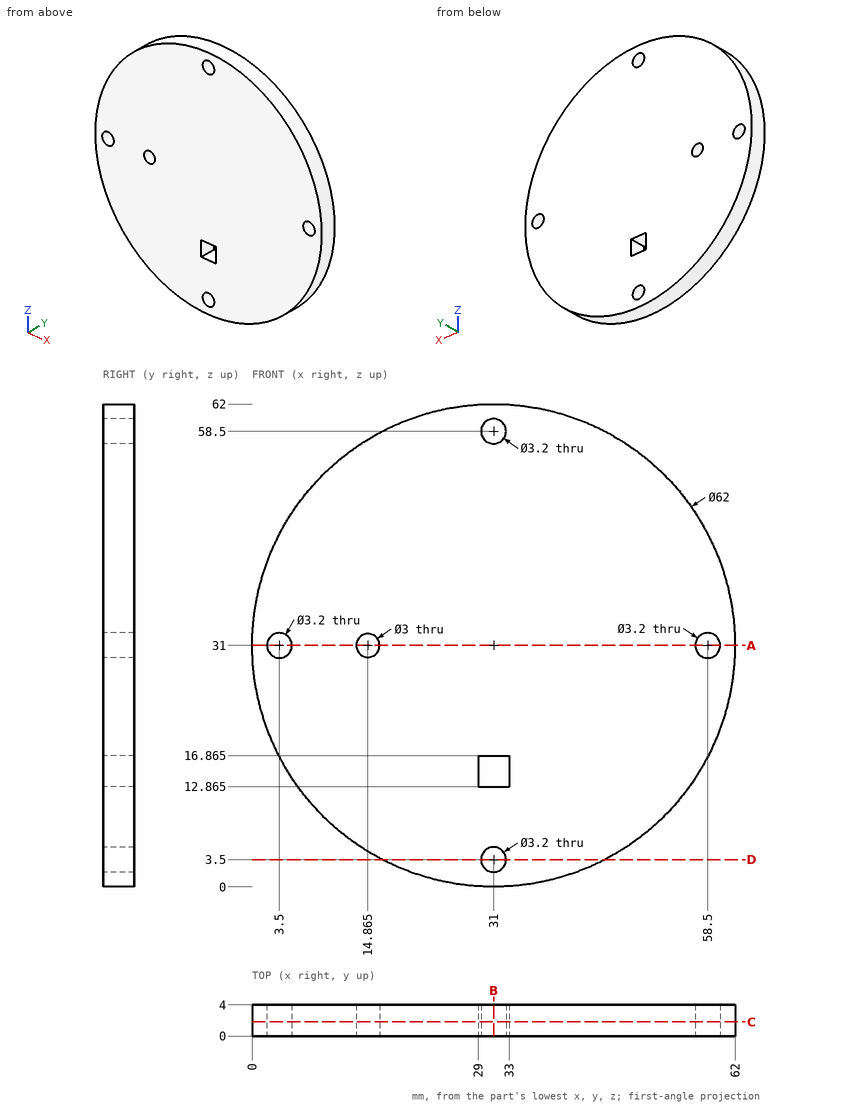
The drawing under review shows one solid part. Ordinate dimensions are in mm from its lowest x, y, z. Give positions to 0.01 mm unless a question says otherwise; leave off trailing zeros. Write each loop counter-clockwise with the first axis right and the second up, starting at its lowest first coordinate (ties: lowest second). Pieces come first, ordered by that corner, then holes.
1. Add section C-C, the plane y = 1.8. Write out the cut boundary in (x, z) (3 decimals).
2. Add section A-A, the plane z = 31. Write out the cut boundary in (x, y) (3 decimals).
3. Add section B-B, the plane x = 31. Write out the cut boundary in (y, z) (3 decimals).
4. Wall thickness on L1, parallel to X at y = 2.9, z = 31 (3 decimals); L2, parallel to X at y = 0.6, z = 16; L3, parallel to Z at x = 3.5, y = 1.45: over which ranges is each line inside the solid? List them lowest first.
5. Add section D-D, the plane z = 3.5. Write out the cut boundary in (x, y), plus the area to 3 significant figures.
6. For P1, Ø1, axis at x = 51.5, y = 3, coming from the -Z side; P2, Ø3, axis at x = 31, z = 58.5, coming from the +Y side; P3, Ø1.2, axis at x = 32, y = 1.5, coming from the +Z side; P4, Ø1, axis at x = 22, y = 3, coming from the -Z side, all flat-tipped, find the tip position at first contact; note any pin that passes through.
Worked answers:
1. outline: circle Ø62 at (31, 31); hole circle Ø3.2 at (3.5, 31); hole circle Ø3 at (14.865, 31); hole (29, 12.865) - (33, 12.865) - (33, 16.865) - (29, 16.865) - close; hole circle Ø3.2 at (31, 3.5); hole circle Ø3.2 at (31, 58.5); hole circle Ø3.2 at (58.5, 31)
2. outline: (0, 0) - (1.9, 0) - (1.9, 4) - (0, 4) - close; (5.1, 0) - (13.365, 0) - (13.365, 4) - (5.1, 4) - close; (16.365, 0) - (56.9, 0) - (56.9, 4) - (16.365, 4) - close; (60.1, 0) - (62, 0) - (62, 4) - (60.1, 4) - close
3. outline: (0, 0) - (4, 0) - (4, 1.9) - (0, 1.9) - close; (0, 5.1) - (4, 5.1) - (4, 12.865) - (0, 12.865) - close; (0, 16.865) - (4, 16.865) - (4, 56.9) - (0, 56.9) - close; (0, 60.1) - (4, 60.1) - (4, 62) - (0, 62) - close
4. L1: x = 0 to 1.9, 5.1 to 13.365, 16.365 to 56.9, 60.1 to 62
4. L2: x = 3.87 to 29, 33 to 58.13
4. L3: z = 16.69 to 29.4, 32.6 to 45.31
5. outline: (16.69, 0) - (29.4, 0) - (29.4, 4) - (16.69, 4) - close; (32.6, 0) - (45.31, 0) - (45.31, 4) - (32.6, 4) - close
5. area: 102 mm2
6. P1: stops at z = 7.31
6. P2: passes through
6. P3: stops at z = 62
6. P4: stops at z = 1.19
